Geometry: final body of the model. Coordinates: model frame, mm. Face numbers are marked on the shaded views. A direction names the side the tool comes from. Round coordinates to 2 decimals unless told otherwise and drop trailing zeros. Write each loop counter-clockwise with the first axis right and the second up, starting at its lowest first coordinate (ties: lowest second). Pieces come first, ordered by that corner, then holes. Notation, with made-up numbers: M -25.75,75.25 L 2.25,75.25 A26 cw 2.25,113.25 Z; hole C 61,55 d5. An arc over 180 degrees is marked long. Use one line per item in the form item = value. Start each with the question number.
Item 1: Section query B-B (x = 2.15). Return loops of the section in (y, z), and give its area (3 significant figures).
Item 2: Pin query (flat end, axial travel): pin 1 Ø1 at (y, z) = (-3, -3.5) entering from +X. Return the tip coordinate at first contact, or that it passes through.
Item 3: Ray query, probe 1 along Y at (x, z) = (1.35, 0); probe 2 along Z at (x, y) = (1.8, 1.5); probe 3 along Z at (x, y) = (3.85, 1.25). Return the intervals inside material, ascending.
Item 4: Section query A-A (x = 2.8). Return loops of the section in (y, z).
Item 5: Pull-direction query (Z, two-part tool) for the marked faces 1 and 2; classes: pulls with the +Z half, pulls with the -Z half, needs draft (parallel to the pull), parting line crosses it, or undercut.
Item 6: Reachability of the marked faces 3, 4, 5 and 6 from +Z, -Z, +X, -X, +Y, -Y: full face, straight path, thin tool, end or side. Return the list, or none.
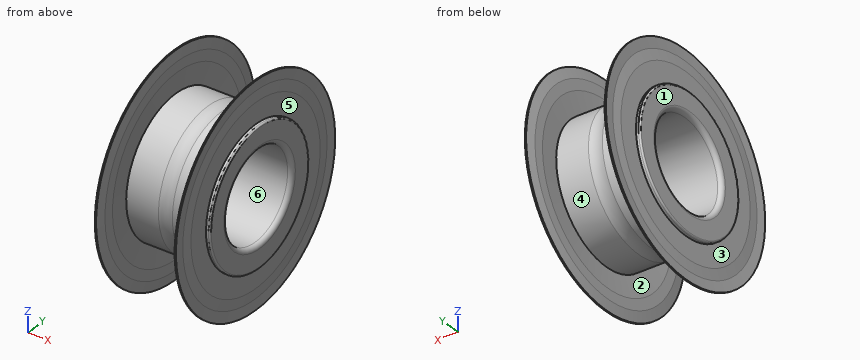
from build123d import *


with BuildPart() as part:
    # Sketch1 → Revolução1 (revolve)
    with BuildSketch(Plane.XY, mode=Mode.PRIVATE) as revolu_o1_sk:
        with BuildLine():
            Line((0, 2.983333333), (0, 2.2))
            ThreePointArc((0, 2.2), (0.058578644, 2.058578644), (0.2, 2))
            Line((0.2, 2), (3.8, 2))
            ThreePointArc((3.8, 2), (3.941421356, 2.058578644), (4, 2.2))
            Line((4, 2.2), (4, 2.983333333))
            ThreePointArc((4, 2.983333333), (3.980473785, 3.030473785), (3.933333333, 3.05))
            Line((3.933333333, 3.05), (2.3122499, 3.05))
            ThreePointArc((2.3122499, 3.05), (2, 3), (1.6877501, 3.05))
            Line((1.6877501, 3.05), (0.066666667, 3.05))
            ThreePointArc((0.066666667, 3.05), (0.019526215, 3.030473785), (0, 2.983333333))
        make_face()
    revolve(revolu_o1_sk.sketch.rotate(Axis((50, 0, 0), (-1, 0, 0)), 270), axis=Axis((50, 0, 0), (-1, 0, 0)))

    # Sketch2 → Revolução2 (revolve)
    with BuildSketch(Plane.XY, mode=Mode.PRIVATE) as revolu_o2_sk:
        Polygon((0.18, 4.9), (0.21, 4.4375), (0.18, 3.975), (0.18, 3.05), (0.24, 3.05), (0.3, 3.975), (0.3, 4.4375), (0.24, 4.9), align=None)
    revolve(revolu_o2_sk.sketch.rotate(Axis((50, 0, 0), (-1, 0, 0)), 270), axis=Axis((50, 0, 0), (-1, 0, 0)))

    # Sketch3 → Revolução3 (revolve)
    with BuildSketch(Plane.XY, mode=Mode.PRIVATE) as revolu_o3_sk:
        Polygon((3.7, 4.4375), (3.7, 3.975), (3.76, 3.05), (3.82, 3.05), (3.82, 3.975), (3.79, 4.4375), (3.82, 4.9), (3.76, 4.9), align=None)
    revolve(revolu_o3_sk.sketch.rotate(Axis((50, 0, 0), (-1, 0, 0)), 270), axis=Axis((50, 0, 0), (-1, 0, 0)))


solid = part.part
Working result:
q1.outline = C 0,0 d6.02; hole C 0,0 d4
q1.area = 15.9 mm²
q2.pin_1 = 3.82
q3.probe_1 = -3.05 to -2, 2 to 3.05
q3.probe_2 = -2.62 to -1.32, 1.32 to 2.62
q3.probe_3 = -2.78 to -1.57, 1.57 to 2.78
q4.outline = C 0,0 d6.1; hole C 0,0 d4
q5.face_1 = needs draft
q5.face_2 = undercut
q6.face_3 = -X
q6.face_4 = none
q6.face_5 = +X
q6.face_6 = +X, -X
